The figure shows three views and two pictorial views of one solid part (mm, origin at its lowest corner). Answer the questions. Round coordinates to 2 decimals unless told otherwise and drop trailing zeros. Loops run counter-clockwise (first coordinate to the right, second up) from the corner with the lowest first, then second, coordinate; pieces in that order, holes last. Notation, with made-up numbers: (84.25, 6.25) -> (141.25, 6.25) arc R25 ccw to (141.25, 28.25) -> close; hole circle Ø5 at (-20, 13). An arc over 180 degrees is marked (long way). Put each result on its own line as item: value.
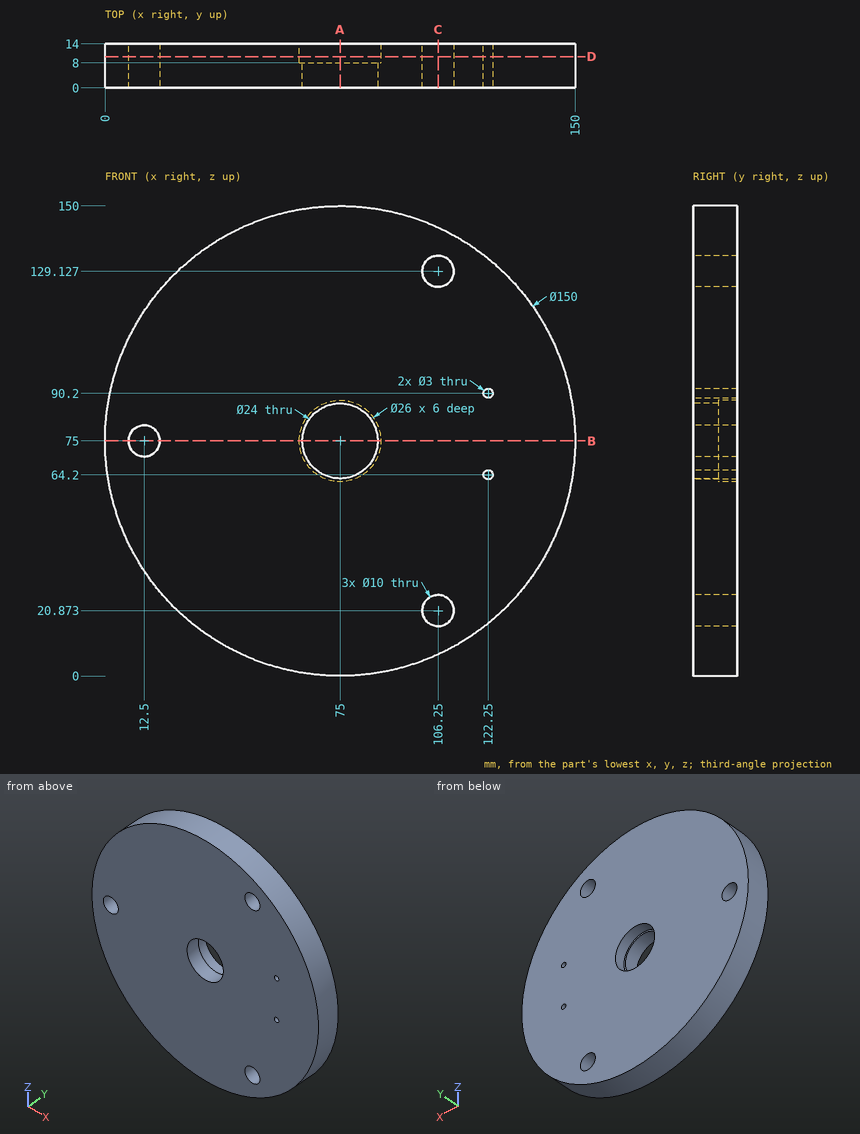
Item 1: The part is cut by section A-A (x = 75). Determine the outline of the cut face in (y, z), then the cut area to 3 significant figures.
Derived:
outline: (0, 0) -> (14, 0) -> (14, 62) -> (8, 62) -> (8, 63) -> (0, 63) -> close; (0, 87) -> (8, 87) -> (8, 88) -> (14, 88) -> (14, 150) -> (0, 150) -> close
area: 1,750 mm^2
Item 2: Find the intervals of material crossed by line 1 along Z through (x, y) = (75, 5.25); line 2 along Z through (x, y) = (75, 9.4); line 3 along X through (y, z) = (4, 72), in increasing order.
Derived:
line 1: z = 0 to 63, 87 to 150
line 2: z = 0 to 62, 88 to 150
line 3: x = 0.06 to 8.5, 16.5 to 63.38, 86.62 to 149.94
Item 3: The part is cut by section B-B (z = 75). Determine the outline of the cut face in (x, y), then the cut area to 3 significant figures.
Derived:
outline: (0, 0) -> (7.5, 0) -> (7.5, 14) -> (0, 14) -> close; (17.5, 0) -> (63, 0) -> (63, 8) -> (62, 8) -> (62, 14) -> (17.5, 14) -> close; (87, 0) -> (150, 0) -> (150, 14) -> (88, 14) -> (88, 8) -> (87, 8) -> close
area: 1,610 mm^2
Item 4: Flat-ended cylindrical pins translate along their axes: pin 1 Ø2.5 at (x, z) = (122.25, 90.2) entering from +Y; pin 2 Ø1.5 at (x, y) = (100.5, 8.5) entering from -Z; pin 3 Ø5 at (x, y) = (49, 5.5) entering from +Z; pin 4 Ø4 at (x, y) = (51.5, 2.5) entering from -Z. Find the tip coordinate at first contact, or state that the pin passes through.
Derived:
pin 1: passes through
pin 2: stops at z = 4.2
pin 3: stops at z = 146.22
pin 4: stops at z = 3.15
Item 5: The part is cut by section C-C (x = 106.25). Determine the outline of the cut face in (y, z), then the cut area to 3 significant figures.
Derived:
outline: (0, 6.82) -> (14, 6.82) -> (14, 15.87) -> (0, 15.87) -> close; (0, 25.87) -> (14, 25.87) -> (14, 124.13) -> (0, 124.13) -> close; (0, 134.13) -> (14, 134.13) -> (14, 143.18) -> (0, 143.18) -> close
area: 1,630 mm^2
Item 6: The part is cut by section D-D (y = 10). Determine the outline of the cut face in (x, z), then the cut area to 3 significant figures.
Derived:
outline: circle Ø150 at (75, 75); hole circle Ø10 at (12.5, 75); hole circle Ø26 at (75, 75); hole circle Ø10 at (106.25, 20.87); hole circle Ø10 at (106.25, 129.13); hole circle Ø3 at (122.25, 64.2); hole circle Ø3 at (122.25, 90.2)
area: 16,900 mm^2
